from build123d import *

# Parameters (mm, degrees)
BOSS_EXTRUDE1_DEPTH     = 55
SKETCH2_W               = 12.5
SKETCH2_H               = 55
CUT_EXTRUDE1_DEPTH      = 10
SKETCH4_R               = 9.45
CUT_EXTRUDE2_DEPTH      = 56
SKETCH5_R               = 9.45
CUT_EXTRUDE3_DEPTH      = 56
SKETCH7_R               = 1.25
CUT_EXTRUDE5_DEPTH      = 35
SKETCH8_R               = 11
CUT_EXTRUDE6_DEPTH      = 35
SKETCH9_R               = 4
CUT_EXTRUDE7_DEPTH      = 1
CUT_EXTRUDE7_DEPTH_BACK = 101
SKETCH11_R              = 4
CUT_EXTRUDE8_DEPTH      = 100
SKETCH12_W              = 0.5
SKETCH12_H              = 7.437726557
SKETCH12_H_2            = 9.137996941
CUT_EXTRUDE9_DEPTH      = 56
SKETCH13_R              = 6.5
CUT_EXTRUDE10_DEPTH     = 56


with BuildPart() as part:
    # Sketch1 → Boss-Extrude1 (new body)
    with BuildSketch(Plane(origin=(0, 0, 0), x_dir=(1, 0, 0), z_dir=(0, 1, 0))):
        Polygon((-37.5, 35), (-50, 35), (-50, -35), (50, -35), (50, 35), (37.5, 35), (37.5, -4), (-37.5, -4), align=None)
    extrude(amount=BOSS_EXTRUDE1_DEPTH)

    # Sketch2 → Cut-Extrude1 (cut)
    with BuildSketch(Plane(origin=(0, 0, -35), x_dir=(-1, 0, 0), z_dir=(0, 0, -1))):
        with Locations((43.75, 27.5)):
            Rectangle(SKETCH2_W, SKETCH2_H)
    extrude(amount=-CUT_EXTRUDE1_DEPTH, mode=Mode.SUBTRACT)

    # Sketch4 → Cut-Extrude2 (cut, through all)
    with BuildSketch(Plane(origin=(0, 55, 0), x_dir=(1, 0, 0), z_dir=(0, 1, 0))):
        with Locations((33, -21.25)):
            Circle(SKETCH4_R)
    extrude(amount=-CUT_EXTRUDE2_DEPTH, mode=Mode.SUBTRACT)

    # Sketch5 → Cut-Extrude3 (cut, through all)
    with BuildSketch(Plane(origin=(0, 55, 0), x_dir=(1, 0, 0), z_dir=(0, 1, 0))):
        with Locations((-34, -20)):
            Circle(SKETCH5_R)
    extrude(amount=-CUT_EXTRUDE3_DEPTH, mode=Mode.SUBTRACT)

    # Sketch7 → Cut-Extrude5 (cut)
    with BuildSketch(Plane(origin=(50, 0, 0), x_dir=(0, 0, -1), z_dir=(1, 0, 0))):
        with Locations((29.173129307, 12)):
            Circle(SKETCH7_R)
        with Locations((-1.826870693, 12)):
            Circle(SKETCH7_R)
        with Locations((-1.826870693, 43)):
            Circle(SKETCH7_R)
        with Locations((29.173129307, 43)):
            Circle(SKETCH7_R)
    extrude(amount=-CUT_EXTRUDE5_DEPTH, mode=Mode.SUBTRACT)

    # Sketch8 → Cut-Extrude6 (cut)
    with BuildSketch(Plane(origin=(50, 0, 0), x_dir=(0, 0, -1), z_dir=(1, 0, 0))):
        with Locations((13.673129307, 27.5)):
            Circle(SKETCH8_R)
    extrude(amount=-CUT_EXTRUDE6_DEPTH, mode=Mode.SUBTRACT)

    # Sketch9 → Cut-Extrude7 (cut, two sides)
    with BuildSketch(Plane(origin=(50, 0, 0), x_dir=(0, 0, -1), z_dir=(1, 0, 0))) as cut_extrude7_sk:
        with Locations((13.673129307, 48.4)):
            Circle(SKETCH9_R)
        with Locations((13.673129307, 6.6)):
            Circle(SKETCH9_R)
    extrude(amount=CUT_EXTRUDE7_DEPTH, mode=Mode.SUBTRACT)
    extrude(cut_extrude7_sk.sketch, amount=-CUT_EXTRUDE7_DEPTH_BACK, mode=Mode.SUBTRACT)

    # Sketch11 → Cut-Extrude8 (cut)
    with BuildSketch(Plane(origin=(-37.5, 0, 0), x_dir=(0, 0, -1), z_dir=(1, 0, 0))):
        with Locations((13.673129307, 27.5)):
            Circle(SKETCH11_R)
    extrude(amount=-CUT_EXTRUDE8_DEPTH, mode=Mode.SUBTRACT)

    # Sketch12 → Cut-Extrude9 (cut, through all)
    with BuildSketch(Plane.XZ):
        with Locations((33.471458783, 32.290249866)):
            Rectangle(SKETCH12_W, SKETCH12_H)
        with Locations((-34.014056432, 31.597087229)):
            Rectangle(SKETCH12_W, SKETCH12_H_2)
    extrude(amount=-CUT_EXTRUDE9_DEPTH, mode=Mode.SUBTRACT)

    # Sketch13 → Cut-Extrude10 (cut, through all)
    with BuildSketch(Plane(origin=(0, 55, 0), x_dir=(1, 0, 0), z_dir=(0, 1, 0))):
        with Locations((3.925383248, -19)):
            Circle(SKETCH13_R)
    extrude(amount=-CUT_EXTRUDE10_DEPTH, mode=Mode.SUBTRACT)


solid = part.part
Geometry check sheet. Reference: the model listing, model coordinates, mm. A direction names the side the tool comes from. Coordinates: 2 decimals unless noted, no trailing zeros. Loops run counter-clockwise (first coordinate to the right, second up) from the corner with the lowest first, then second, coordinate; pieces in that order, holes last. Notation, with made-up numbers: (2.25, -34.5) - (54.25, -34.5) arc R16 ccw to (54.25, -28.5) - close; hole circle Ø10 at (35.5, -23). An arc over 180 degrees is marked (long way). Use one line per item in the form item = value. Start each with the question number.
Item 1: Section check D-D, the plane z = 2. Enter the section's corners in (x, y), and give its area (3 significant figures).
Item 2: Section check C-C, the plane x = 26. Enter the section's corners in (y, z).
Item 3: Mould release check, pull along Y, two halves, no side actions. Record for faces 4 (the face through (-1, 55, 7)), 5 (the face through (43.838, 44.495, -12.806)), 6 (the face through (-43.662, 6.776, -9.677)), 7 (the face through (-34.264, 27, 32)): +Y half, -Y half, draft (parallel to the pull), parting line (faces both ways), or undercut.
Item 4: Tool access check on faces 1 (the face through (43.84, 13.24, 1.99)), 2 (the face through (-33.764, 27, 32)), 3 (the face through (1, 27, 4)). Record the directions out of +Z, -Z, +X, -X, +Y, -Y that give a thin tool (end or side, any length) a straight path to the whole face; none if there is none.
Item 5: Thickness scan on probe 1 along Z at (x, y) = (33, 25); probe 2 along Z at (x, y) = (4, 29); probe 3 along X at (y, z) = (14, -1). Record the ranges inside material, lowest first.
Item 6: Gauge pin test, flat ends, axial feed: pin 1 (10.5 mm diameter, centred on y = 6.6, z = -13.67, fed in from -X); pin 2 (4 mm diameter, centred on x = -38, y = 49.5, fed in from -Z); pin 3 (1.5 mm diameter, centred on x = 12.5, y = 29, fed in from -Z); pin 4 (13 mm diameter, centred on y = 27.5, z = -13.67, fed in from +X). Record the tip position at first contact, or that the pin passes through.
Item 7: Section check B-B, the plane y = 21.5. Enter the section's corners in (x, z).
Item 8: Section check A-A, the plane y = 6.6. Enter the section's corners in (x, z).
Computed:
q1.outline = (-50, 0) - (-37.5, 0) - (-37.5, 55) - (-50, 55) - close; (37.5, 0) - (50, 0) - (50, 10.76) - (37.5, 10.76) - close; (37.5, 13.24) - (50, 13.24) - (50, 41.76) - (37.5, 41.76) - close; (37.5, 44.24) - (50, 44.24) - (50, 55) - (37.5, 55) - close
q1.area = 1,310 mm2
q2.outline = (0, 4) - (55, 4) - (55, 14.9) - (0, 14.9) - close; (0, 27.6) - (55, 27.6) - (55, 35) - (0, 35) - close
q3.face_4 = +Y half
q3.face_5 = undercut
q3.face_6 = undercut
q3.face_7 = draft
q4.face_1 = +X
q4.face_2 = +Z, +Y, -Y
q4.face_3 = -Z, +Y, -Y
q5.probe_1 = 4 to 11.8, 30.7 to 35
q5.probe_2 = 4 to 12.5, 25.5 to 35
q5.probe_3 = -50 to -37.5, 37.5 to 50
q6.pin_1 = -50
q6.pin_2 = -25
q6.pin_3 = 4
q6.pin_4 = -37.5
q7.outline = (-50, -25) - (-37.5, -25) - (-37.5, 4) - (37.5, 4) - (37.5, -4.45) - (50, -4.45) - (50, 35) - (33.72, 35) - (33.72, 30.67) arc R9.45 cw (long way) to (33.22, 30.7) - (33.22, 35) - (-33.76, 35) - (-33.76, 29.45) arc R9.45 cw (long way) to (-34.26, 29.45) - (-34.26, 35) - (-50, 35) - close; (37.5, -35) - (50, -35) - (50, -22.89) - (37.5, -22.89) - close; hole circle Ø13 at (3.93, 19)
q8.outline = (-50, -25) - (-37.5, -25) - (-37.5, -17.67) - (-50, -17.67) - close; (-50, -9.67) - (-37.5, -9.67) - (-37.5, 4) - (37.5, 4) - (37.5, -9.67) - (50, -9.67) - (50, 35) - (33.72, 35) - (33.72, 30.67) arc R9.45 cw (long way) to (33.22, 30.7) - (33.22, 35) - (-33.76, 35) - (-33.76, 29.45) arc R9.45 cw (long way) to (-34.26, 29.45) - (-34.26, 35) - (-50, 35) - close; (37.5, -35) - (50, -35) - (50, -17.67) - (37.5, -17.67) - close; hole circle Ø13 at (3.93, 19)
